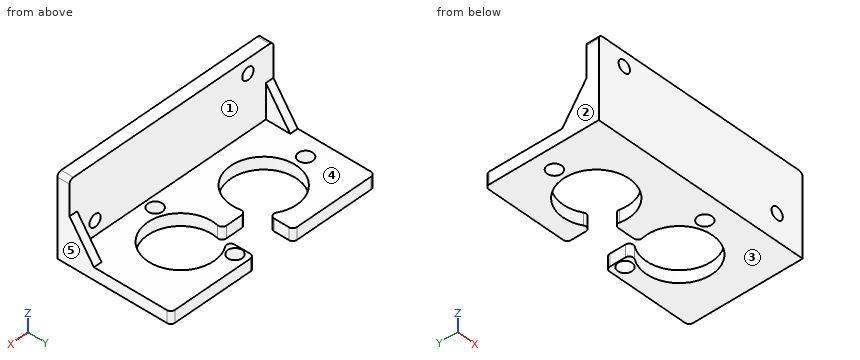
Autodesk Fusion 360 part; units mm, degrees
sketch "Sketch1" plane through (0, 0, 0) normal (0, 1, 0) x (1, 0, 0)
  line L0 (0, 0) -> (-54, 0)
  line L1 (-54, 0) -> (-54, -20)
  line L2 (-54, -20) -> (0, -20)
  line L3 (0, -20) -> (0, 0)
  dimension "d5" = 54
  dimension "d6" = 20
extrude "Extrude1" add sketch "Sketch1" along normal blind 3
sketch "Sketch2" plane through (0, 3, 0) normal (0, 1, 0) x (-1, 0, 0)
  line L0 (0, 20) -> (0, 0)
  line L1 (0, 0) -> (54, 0)
  line L2 (54, 0) -> (54, 20)
  line L3 (54, 20) -> (0, 20)
  line L4 (0, 0) -> (54, 0)
  line L5 (54, 0) -> (54, 3)
  line L6 (54, 3) -> (0, 3)
  line L7 (0, 3) -> (0, 0)
  dimension "d9" = 3
extrude "Extrude2" add sketch "Sketch2" along normal blind 25 contours L0 L1 L2 L4 L5 L6 L7
sketch "Sketch3" plane through (0, 3, 0) normal (0, 1, 0) x (-1, 0, 0)
  line L0 (0, 3) -> (54, 3)
  line L1 (54, 3) -> (54, 20)
  line L2 (54, 20) -> (0, 20)
  line L3 (0, 20) -> (0, 3)
  circle A0 centre (6.75, 6.5) radius 1.5
  circle A1 centre (47.25, 16.5) radius 1.5
  line L4 (6.75, 16.5) -> (47.25, 16.5) construction
  line L5 (47.25, 16.5) -> (47.25, 6.5) construction
  line L6 (47.25, 6.5) -> (6.75, 6.5) construction
  line L7 (6.75, 6.5) -> (6.75, 16.5) construction
  line L8 (6.75, 16.5) -> (47.25, 6.5) construction
  line L9 (47.25, 16.5) -> (6.75, 6.5) construction
  line L10 (0, 20) -> (54, 3) construction
  line L11 (54, 20) -> (0, 3) construction
  point P0 (27, 11.5)
  point P1 (27, 11.5)
  dimension "d12" = 10
  dimension "d13" = 40.5
  dimension "d16" = 3
  dimension "d17" = 3
extrude "Extrude3" cut sketch "Sketch3" against normal up to surface (3 mm away) contours A0 | A1
sketch "Sketch4" plane through (0, 0, 0) normal (0, 0, -1) x (-1, 0, 0)
  line L0 (0, 0) -> (54, 0)
  line L1 (54, 0) -> (54, 28)
  line L2 (54, 28) -> (0, 28)
  line L3 (0, 28) -> (0, 0)
  line L4 (2, 28) -> (52, 28) construction
  line L5 (52, 28) -> (52, 3) construction
  line L6 (52, 3) -> (2, 3) construction
  line L7 (2, 3) -> (2, 28) construction
  circle A0 centre (20, 5.5) radius 1.75
  circle A1 centre (49.085, 15.5) radius 1.75
  line L8 (2, 15.5) -> (52, 15.5) construction
  line L9 (22.016, 28) -> (32.316, 28)
  line L10 (32.316, 28) -> (32.316, 21.3408)
  line L11 (30.3834, 18.4) -> (23.6166, 18.4)
  line L12 (22.016, 20.9982) -> (22.016, 28)
  circle A2 centre (20.062, 25.085) radius 1.75
  arc A3 (22.016, 20.9982) -> (23.6166, 18.4) centre (16, 15.5) ccw
  arc A4 (30.3834, 18.4) -> (32.316, 21.3408) centre (38, 15.5) ccw
  point P0 (27, 28)
  dimension "d20" = 50
  dimension "d21" = 25
  dimension "d24" = 18
  dimension "d25" = 2.5
  dimension "d26" = 3.5
  dimension "d27" = 3.5
  dimension "d28" = 2.915
  dimension "d29" = 12.5
  dimension "d30" = 16.3
  dimension "d31" = 16.3
  dimension "d33" = 14
  dimension "d34" = 14
  dimension "d35" = 20.016
  dimension "d36" = 9.6
  dimension "d37" = 3.5
  dimension "d38" = 2.915
  dimension "d39" = 18.062
  dimension "d40" = 10.3
extrude "Extrude4" cut sketch "Sketch4" against normal up to surface (3 mm away) contours L2 L9 L10 L11 L12 A3 A4 | A0 | A1 | A2
sketch "Sketch5" plane through (-54, 0, 0) normal (-1, 0, 0) x (0, 0, 1)
  line L0 (0, 0) -> (20, 0)
  line L1 (20, 0) -> (20, 3)
  line L2 (20, 3) -> (3, 3)
  line L3 (3, 3) -> (3, 28)
  line L4 (3, 28) -> (0, 28)
  line L5 (0, 28) -> (0, 0)
  line L6 (3, 9) -> (11.5, 3)
  dimension "d46" = 6
extrude "Extrude5" add sketch "Sketch5" against normal blind 2 contours L2 L3 L6
ref_plane "WorkPlane1" through (-27, 14, 10) normal (-1, 0, 0) x (0, 0, 1)
fillet "Fillet1" radius 1 10 edges at (-54, 28, 1.5) (-54, 1.5, 20) (-32.316, 28, 1.5) (-32.316, 21.3408, 1.5) (-30.3834, 18.4, 1.5) (-23.6166, 18.4, 1.5) (-22.016, 20.9982, 1.5) (-22.016, 28, 1.5) (0, 28, 1.5) (0, 1.5, 20)
mirror "Mirror1" about plane through (-27, 14, 10) normal (-1, 0, 0) of "Extrude5"
equation "height_base = 20 mm"
equation "width = 54 mm"
equation "thick = 3 mm"
equation "height_sensor = 25 mm"
equation "d5 = width"
equation "d6 = height_base"
equation "d7 = thick"
equation "d9 = thick"
equation "d10 = height_sensor"
equation "d12 = height_base * 1 / 2"
equation "d13 = width * 3 / 4"
equation "screw_base = 3 mm"
equation "screw_sensor = 3.5 mm"
equation "d16 = screw_base"
equation "d17 = screw_base"
equation "d26 = screw_sensor"
equation "d27 = screw_sensor"
equation "d30 = sensor"
equation "d31 = sensor"
equation "sensor = 16.3 mm"
equation "d37 = screw_sensor"
equation "fillet = 1 mm"
equation "d51 = fillet"
Geometry check sheet. Reference: the model listing, model coordinates, mm. Face numbers are marked on the shaded views. A direction names the side the tool comes from. Give positions to 0.01 mm unless a question says otherwise; leave off trailing zeros. Order: outer loops, then holes, each group sorted by start corner. A loop starts at its lowest first (then second) coordinate and runs counter-clockwise, first axis right, second up. Notation, with made-up numbers: (65.25, -8.75) -> (90.25, -8.75) arc R34 ccw to (90.25, 27.25) -> close; hole circle Ø7 at (-16.5, 53.5). An arc over 180 degrees is marked (long way). Write each question's results on one line, items separated by ' | '. Start each with the question number.
(1) Access from +Z, -Z, +X, -X, +Y, -Y to the whole of each face (thin tool, end or side, straight path). Record for the marked faces 4 and 5.
(2) Sectioned sample at B-B (z = 16.5). Enter the section's corners in (x, y), plus the area to 3 significant figures.
(3) Mould release check, pull along X, two halves, no side actions. Record for the marked faces 1, 2 and 3: pulls with the +X half, pulls with the -X half, needs draft (parallel to the pull), parting line crosses it, or undercut.
(4) Sectioned sample at A-A (x = -6.75). Enter the section's corners in (y, z), plus the area to 3 significant figures.
(5) Scan lines: line 1 (Z direction, x = -6.75, y = 1.4); line 2 (Y direction, x = -20, z = 1.4); line 3 (X direction, y = 3.25, z = 4.25). Record each from-to range of solid material in increasing order.
(6) Sectioned sample at C-C (y = 5.5). Enter the section's corners in (x, z), plus the area to 3 significant figures.
(7) Gauge pin test, flat ends, axial feed: P1, Ø5, axis at x = -47.25, z = 16.5, coming from the +Y side; P2, Ø5.5, axis at x = -49.085, y = 15.5, coming from the +Z side; P3, Ø6.5, axis at y = 5.5, z = 7, coming from the +X side; P4, Ø2.5, axis at x = -27.5, z = 1, coming from the +Y side. Record the tip position at first contact, or that the pin passes through.
(8) Sectioned sample at D-D (y = 16.5). Enter the section's corners in (x, z), plus the area to 3 significant figures.
Answer below:
1) face 4: +Z, +Y | face 5: +Z, -Z, +X, +Y, -Y
2) outline: (-54, 0) -> (-48.75, 0) -> (-48.75, 3) -> (-54, 3) -> close; (-45.75, 0) -> (0, 0) -> (0, 3) -> (-45.75, 3) -> close | area: 153 mm2
3) face 1: undercut | face 2: pulls with the -X half | face 3: needs draft
4) outline: (0, 0) -> (28, 0) -> (28, 3) -> (3, 3) -> (3, 5) -> (0, 5) -> close; (0, 8) -> (3, 8) -> (3, 20) -> (0, 20) -> close | area: 126 mm2
5) line 1: 0 to 5, 8 to 20 | line 2: 0 to 3.75, 7.25 to 8.4, 22.6 to 23.34, 26.83 to 28 | line 3: -54 to -52, -2 to 0
6) outline: (-54, 0) -> (-21.75, 0) -> (-21.75, 3) -> (-52, 3) -> (-52, 7.96) -> (-54, 7.96) -> close; (-18.25, 0) -> (0, 0) -> (0, 7.96) -> (-2, 7.96) -> (-2, 3) -> (-18.25, 3) -> close | area: 171 mm2
7) P1: y = 3 | P2: z = 3 | P3: x = 0 | P4: y = 18.4
8) outline: (-54, 0) -> (-50.52, 0) -> (-50.52, 3) -> (-54, 3) -> close; (-47.65, 0) -> (-46.09, 0) -> (-46.09, 3) -> (-47.65, 3) -> close; (-29.91, 0) -> (-24.09, 0) -> (-24.09, 3) -> (-29.91, 3) -> close; (-7.91, 0) -> (0, 0) -> (0, 3) -> (-7.91, 3) -> close | area: 56.3 mm2
